```python
from build123d import *

# Parameters (mm, degrees)
SKETCH1_W           = 63.5
SKETCH1_H           = 12.7
SKETCH1_R           = 1.5875
BOSS_EXTRUDE1_DEPTH = 3
FILLET1_R           = 6.35


with BuildPart() as part:
    # Sketch1 → Boss-Extrude1 (new body)
    with BuildSketch(Plane(origin=(0, 0, 0), x_dir=(1, 0, 0), z_dir=(0, 1, 0))):
        Rectangle(SKETCH1_W, SKETCH1_H)
        with Locations(Location((-12.7, 0, 0), (0, 0, 270))):
            Circle(SKETCH1_R, mode=Mode.SUBTRACT)
        with Locations(Location((12.7, 0, 0), (0, 0, 270))):
            Circle(SKETCH1_R, mode=Mode.SUBTRACT)
        with Locations(Location((25.4, 0, 0), (0, 0, 270))):
            Circle(SKETCH1_R, mode=Mode.SUBTRACT)
        with Locations(Location((-25.4, 0, 0), (0, 0, 270))):
            Circle(SKETCH1_R, mode=Mode.SUBTRACT)
    extrude(amount=BOSS_EXTRUDE1_DEPTH)

    # Fillet1
    fillet1_edges = [part.edges().sort_by_distance(p)[0] for p in [
        (-31.75, 1.5, -6.35),
        (-31.75, 1.5, 6.35),
        (31.75, 1.5, -6.35),
        (31.75, 1.5, 6.35),
    ]]
    fillet(fillet1_edges, radius=FILLET1_R - 0.0001)  # a hair under: the kernel refuses the full size


solid = part.part
```
Verification items for the finished model (mm, model axes). Coordinates: 2 decimals unless noted, no trailing zeros. Order: outer loops, then holes, each group sorted by start corner. A loop starts at its lowest first (then second) coordinate and runs counter-clockwise, first axis right, second up. Notation, with made-up numbers: (79.5, 6) -> (117.5, 6) arc R23 ccw to (117.5, 16) -> close; hole circle Ø8 at (67, 45.5). An arc over 180 degrees is marked (long way). Answer as CSV lines item,"result". Start each with the question number.
1) Cross-section at B-B, the plane y = 1.75. Give the number of separate pieces and of enclosed holes in the cut face, then the cut area to 3 significant figures.
2) Release check for a two-part mould opening along X. For faces 1 (the face through (0, 0, 0)), 2 (the face through (-29.94, 1.52, 4.44)), 3 (the face through (14.274, 1.479, -0.207)) record: released by +X, released by -X, zero draft, split by the parting line, or undercut.
3) Material ranges on L1, parallel to X at y = 1.15, z = 0; L2, parallel to X at y = 1.65, z = 0.25; L3, parallel to Z at x = 26.5, y = 1.9, recorded low to high. Write a range as [from, to].
4) Gauge pin test, flat end, axial feed: pin 1 Ø1 at (y, z) = (1, 3) entering from +X. Record the tip position at first contact, or that the pin passes through.
5) Cross-section at A-A, the plane x = 12.7. Record the boundary of the cut face in (y, z).
6) Cross-section at C-C, the plane z = 1. Record the boundary of the cut face in (x, y).
Conclusion:
1,separate pieces,"1"
1,enclosed holes,"4"
1,area,"740 mm²"
2,face 1,"zero draft"
2,face 2,"released by -X"
2,face 3,"undercut"
3,L1,"x = [-31.75, -26.99], [-23.81, -14.29], [-11.11, 11.11], [14.29, 23.81], [26.99, 31.75]"
3,L2,"x = [-31.75, -26.97], [-23.83, -14.27], [-11.13, 11.13], [14.27, 23.83], [26.97, 31.75]"
3,L3,"z = [-6.25, -1.14], [1.14, 6.25]"
4,pin 1,"stops at x = 31.24"
5,outline,"(0, -6.35) -> (3, -6.35) -> (3, -1.59) -> (0, -1.59) -> close; (0, 1.59) -> (3, 1.59) -> (3, 6.35) -> (0, 6.35) -> close"
6,outline,"(-31.67, 0) -> (-26.63, 0) -> (-26.63, 3) -> (-31.67, 3) -> close; (-24.17, 0) -> (-13.93, 0) -> (-13.93, 3) -> (-24.17, 3) -> close; (-11.47, 0) -> (11.47, 0) -> (11.47, 3) -> (-11.47, 3) -> close; (13.93, 0) -> (24.17, 0) -> (24.17, 3) -> (13.93, 3) -> close; (26.63, 0) -> (31.67, 0) -> (31.67, 3) -> (26.63, 3) -> close"
